Geometry: final body of the model. Coordinates: model frame, mm. A direction names the side the tool comes from. Coordinates: 2 decimals unless noted, no trailing zeros. Order: outer loops, then holes, each group sorted by start corner. A loop starts at its lowest first (then second) coordinate and runs counter-clockwise, first axis right, second up. Notation, with made-up numbers: (-17, 5.25) -> (-3, 5.25) arc R23 cw to (-3, 30.25) -> close; hole circle Ø5 at (80, 15.5). An arc over 180 degrees is marked (long way). Answer in a Markdown table with one row per item. Add a question column.
1) Section query D-D on z = -57. Return the cut outline in (x, y), then the cut area to 3 significant figures.
2) Section query B-B on x = -7. Return the cut outline in (y, z) (1 decimal).
3) Set-up query: faces 1 (the face through (-20, -10, -25)), 2 (the face through (15, -17, -60)), 3 (the face through (22, -27, -60)), 4 (the face through (-14.985, -22.465, 0.66)). Return all of +Z, -Z, +X, -X, +Y, -Y with unobstructed straight access to the full face (end or side cutting, diameter ignored); none if empty.
4) Contact query for flat-ended pins moving along their axis: P1, Ø15, axis at x = 5, z = -35.5, coming from the -Y side; P2, Ø5, axis at y = -16.5, z = -11.5, coming from the +X side; P3, Ø10, axis at x = 19, y = -20.5, coming from the +Z side. Output: stop coordinate, or through.
5) Section query C-C on y = -16.5. Return the cut outline in (x, z), then the cut area to 3 significant figures.
6) Section query A-A on z = -43.5. Return the cut outline in (x, y), then the cut area to 3 significant figures.
7) Ray query, line 1 (X direction, y = -13.5, z = -30.5); line 2 (Z direction, x = -3, y = 22.5); line 3 (Y direction, x = 3, z = -23). Return the intervals inside material, ascending. Write a range as from..to.
```python
from build123d import *

# Parameters (mm, degrees)
F0_R          = 15
F0_W          = 15
F0_H          = 20
F1_DEPTH      = 20
F2_DEPTH      = 45
F3_DEPTH      = 25
F3_DEPTH_BACK = 35
F4_R          = 9.99999
F6_DEPTH      = 25
F7_DEPTH      = 5


# Not quite as in the source:
# - a fillet or chamfer is up to 0.001 mm smaller than in the source, because OpenCascade refuses the exact size


with BuildPart() as f1:
    # F0 (on Front) → F1 (new body)
    with BuildSketch(Plane.XZ):
        with BuildLine():
            ThreePointArc((-20, 0), (0, -20), (20, 0))
            ThreePointArc((20, 0), (19.7144383856, 3.3676281177), (18.8659080861, 6.6390897033))
            ThreePointArc((18.8659080861, 6.6390897033), (-3.3676281177, 19.7144383856), (-20, 0))
        make_face()
        Circle(F0_R, mode=Mode.SUBTRACT)
        with BuildLine():
            ThreePointArc((18.8659080861, 6.6390897033), (19.7144383856, 3.3676281177), (20, 0))
            ThreePointArc((20, 0), (0, -20), (-20, 0))
            Line((-20, 0), (-20, -50))
            Line((-20, -50), (-5, -50))
            Line((-5, -50), (-5, -30))
            Line((-5, -30), (15, -30))
            Line((15, -30), (15, -60))
            Line((15, -60), (30, -60))
            Line((30, -60), (30, -25))
            Line((30, -25), (18.8659080861, 6.6390897033))
        make_face()
        with Locations((22.5, -70)):
            Rectangle(F0_W, F0_H)
    extrude(amount=F1_DEPTH)

    # F0 (on Front) → F2 (join)
    with BuildSketch(Plane.XZ):
        with Locations((22.5, -70)):
            Rectangle(F0_W, F0_H)
    extrude(amount=F2_DEPTH)

    # F0 (on Front) → F3 (join, two sides)
    with BuildSketch(Plane.XZ) as f3_sk:
        Circle(F0_R)
    extrude(amount=F3_DEPTH)
    extrude(f3_sk.sketch, amount=-F3_DEPTH_BACK)

    # F4 (radius 10 in the source; OpenCascade refuses exactly that, so slightly less here)
    f4_edges = [f1.edges().sort_by_distance(p)[0] for p in [
        (22.5, -45, -60),
        (22.5, -45, -80),
    ]]
    fillet(f4_edges, radius=F4_R)

    # F5 (on face) → F6 (join)
    with BuildSketch(Plane(origin=(0, 35, 0), x_dir=(-1, 0, 0), z_dir=(0, 1, 0))):
        with BuildLine():
            Line((30, 15), (0, 15))
            ThreePointArc((0, 15), (10.6066017178, 10.6066017178), (15, 0))
            ThreePointArc((15, 0), (10.6066017178, -10.6066017178), (0, -15))
            Line((0, -15), (45, -15))
            Line((45, -15), (45, 5))
            Line((45, 5), (30, 5))
            Line((30, 5), (30, 15))
        make_face()
    extrude(amount=-F6_DEPTH)

    # F5 (on face) → F7 (cut)
    with BuildSketch(Plane(origin=(0, 35, 0), x_dir=(-1, 0, 0), z_dir=(0, 1, 0))):
        with BuildLine():
            Line((30, 15), (0, 15))
            ThreePointArc((0, 15), (10.6066017178, 10.6066017178), (15, 0))
            ThreePointArc((15, 0), (10.6066017178, -10.6066017178), (0, -15))
            Line((0, -15), (45, -15))
            Line((45, -15), (45, 5))
            Line((45, 5), (30, 5))
            Line((30, 5), (30, 15))
        make_face()
    extrude(amount=-F7_DEPTH, mode=Mode.SUBTRACT)


solid = f1.part
```
Result:
| question | item | result |
|---|---|---|
| 1 | outline | (15, -20) -> (30, -20) -> (30, 0) -> (15, 0) -> close |
| 1 | area | 300 mm2 |
| 2 | outline | (-25, -13.3) -> (-20, -13.3) -> (-20, -50) -> (0, -50) -> (0, -13.3) -> (10, -13.3) -> (10, -15) -> (30, -15) -> (30, -13.3) -> (35, -13.3) -> (35, 13.3) -> (30, 13.3) -> (30, 15) -> (10, 15) -> (10, 13.3) -> (0, 13.3) -> (0, 18.7) -> (-20, 18.7) -> (-20, 13.3) -> (-25, 13.3) -> close |
| 3 | face 1 | +Z, -Z, -X, -Y |
| 3 | face 2 | -Z, +Y, -Y |
| 3 | face 3 | +Z, +X, -X, -Y |
| 3 | face 4 | -Y |
| 4 | P1 | y = -20 |
| 4 | P2 | x = 26.13 |
| 4 | P3 | z = 14.26 |
| 5 | outline | (-20, -50) -> (-5, -50) -> (-5, -30) -> (15, -30) -> (15, -80) -> (30, -80) -> (30, -25) -> (18.87, 6.64) arc R20 ccw to (-20, 0) -> close |
| 5 | area | 3,070 mm2 |
| 6 | outline | (-20, -20) -> (-5, -20) -> (-5, 0) -> (-20, 0) -> close; (15, -20) -> (30, -20) -> (30, 0) -> (15, 0) -> close |
| 6 | area | 600 mm2 |
| 7 | line 1 | -20..-5, 15..30 |
| 7 | line 2 | -15..15 |
| 7 | line 3 | -20..0 |
